Here's the drawing with two shaded views (mm, measured from the low corner). I have some questions. Give positions to 0.01 mm unless a question says otherwise; leave off trailing zeros. Order: outer loops, then holes, each group sorted by start corner. A loop starts at its lowest first (then second) coordinate and runs counter-clockwise, first axis right, second up. Notation, with made-up numbers: M 30,64 L 80,64 A22 ccw 80,75 Z; hole C -35.5,-12.5 d10. An arc over 180 degrees is marked long. Use a Markdown table: item, result. Add a question column.
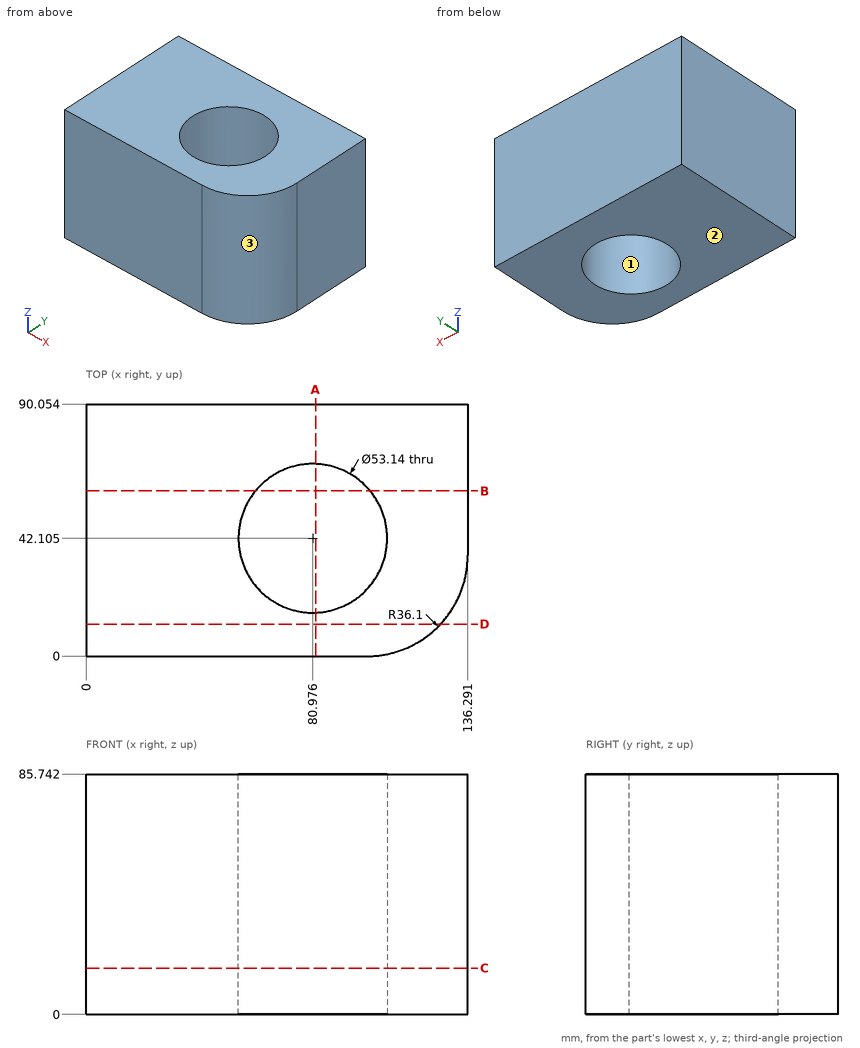
1) Suppose I cut it at D-D on y = 11.5. Please give me the cut outline in (x, z).
2) We'd pull the mould along X, two halves only. Please class the marked faces 1, 2 and 3: pulls with the +X half, pulls with the -X half, needs draft (parallel to the pull), parting line crosses it, or undercut.
3) Suppose I cut it at B-B on y = 59. Please give me the cut outline in (x, z).
4) Please list where these lines run through material, in increasing order: line 1 (X direction, y = 42, z = 61); line 2 (X direction, y = 31, z = 9) (1 decimal); line 3 (Y direction, x = 97, z = 79.5) (1 decimal). Write a range as from..to.
5) Suppose I cut it at C-C on z = 16.5. Please give me the cut outline in (x, y) (1 decimal).
6) For pin 1 (2 mm diameter, centred on y = 28.5, z = 39.5, fed in from +X), with a flat end and sliding along its axis, tell me the tip position at first contact or that it passes through.
7) Suppose I cut it at A-A on x = 82. Please give me the cut outline in (y, z) (1 decimal), and give its area (3 significant figures).
Values found:
| question | item | result |
|---|---|---|
| 1 | outline | M 0,0 L 126.61,0 L 126.61,85.74 L 0,85.74 Z |
| 2 | face 1 | undercut |
| 2 | face 2 | needs draft |
| 2 | face 3 | pulls with the +X half |
| 3 | outline | M 0,0 L 60.47,0 L 60.47,85.74 L 0,85.74 Z; M 101.48,0 L 136.29,0 L 136.29,85.74 L 101.48,85.74 Z |
| 4 | line 1 | x = 0..54.41, 107.55..136.29 |
| 4 | line 2 | x = 0..56.8, 105.1..135.9 |
| 4 | line 3 | y = 0..20.9, 63.3..90.1 |
| 5 | outline | M 0,0 L 100.2,0 A36.1 ccw 136.3,36.1 L 136.3,90.1 L 0,90.1 Z; hole C 81,42.1 d53.1 |
| 6 | pin 1 | stops at x = 135.68 |
| 7 | outline | M 0,0 L 15.6,0 L 15.6,85.7 L 0,85.7 Z; M 68.7,0 L 90.1,0 L 90.1,85.7 L 68.7,85.7 Z |
| 7 | area | 3,170 mm^2 |
